The figure shows three views and two pictorial views of one solid part (mm, origin at its lowest corner). Answer the questions. Give positions to 0.01 mm unless a question says otherwise; leave off trailing zeros. Loops run counter-clockwise (first coordinate to the right, second up) from the corner with the lowest first, then second, coordinate; pieces in that order, holes last. Notation, with made-up numbers: M -7.5,85 L 27.5,85 A13 ccw 27.5,97 Z; hole C -20,17.25 d4. An arc over 180 degrees is marked long. Answer in a Markdown table with one row per item. Add a question column.
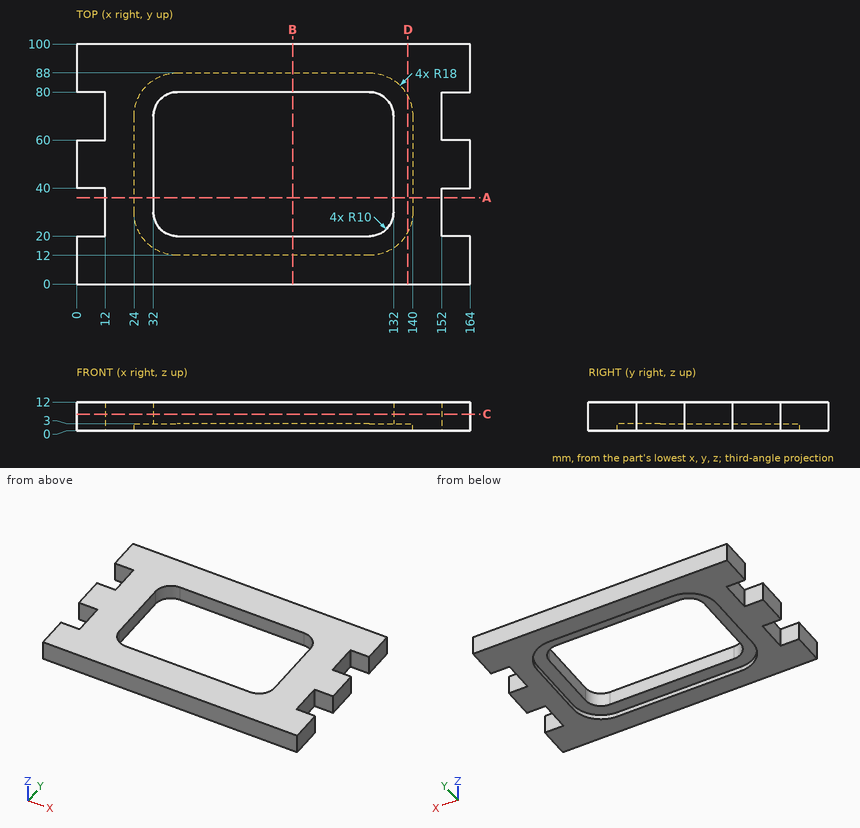
(1) Section B-B, the plane x = 90 is taken. Determine the outline of the cut face in (y, z).
(2) Section A-A, the plane y = 36 is taken. Determine the outline of the cut face in (x, z).
(3) Section D-D, the plane x = 138 is taken. Determine the outline of the cut face in (y, z).
(4) Section C-C, the plane z = 7 is taken. Determine the outline of the cut face in (x, y).
(5) This flat-tipped pin is pushed along its axis until it touches: P1, Ø1.5, axis at x = 67, y = 79, coming from the -Z side. Where does it stop, or does it pass through?
(6) Consider line 1 along Y through (x, z) = (64.5, 5.75); line 2 along X through (y, z) = (49, 9.25); line 3 along X through (y, z) = (63, 9.5). Determine where each line is inside the solid, lowest interval first. Write a range as from..to.
Numbers:
| question | item | result |
|---|---|---|
| 1 | outline | M 0,0 L 12,0 L 12,3 L 20,3 L 20,12 L 0,12 Z; M 80,3 L 88,3 L 88,0 L 100,0 L 100,12 L 80,12 Z |
| 2 | outline | M 12,0 L 24,0 L 24,3 L 32,3 L 32,12 L 12,12 Z; M 132,3 L 140,3 L 140,0 L 152,0 L 152,12 L 132,12 Z |
| 3 | outline | M 0,0 L 21.75,0 L 21.75,3 L 78.25,3 L 78.25,0 L 100,0 L 100,12 L 0,12 Z |
| 4 | outline | M 0,0 L 164,0 L 164,20 L 152,20 L 152,40 L 164,40 L 164,60 L 152,60 L 152,80 L 164,80 L 164,100 L 0,100 L 0,80 L 12,80 L 12,60 L 0,60 L 0,40 L 12,40 L 12,20 L 0,20 Z; hole M 32,30 A10 ccw 42,20 L 122,20 A10 ccw 132,30 L 132,70 A10 ccw 122,80 L 42,80 A10 ccw 32,70 Z |
| 5 | P1 | passes through |
| 6 | line 1 | y = 0..20, 80..100 |
| 6 | line 2 | x = 0..32, 132..164 |
| 6 | line 3 | x = 12..32, 132..152 |
